Geometry: see drawing. Coordinates: mm, zero at the bounding-box minimum. A direction names the side the tool comes from. Coordinates: 2 decimals unless noted, no trailing zeros. Loops run counter-clockwise (first coordinate to the right, second up) from the corner with the lowest first, then second, coordinate; pieces in that order, holes last. Notation, with made-up numbers: (21.25, 64.5) -> (43.25, 64.5) arc R33 cw to (43.25, 103.5) -> close; hole circle Ø8 at (-26, 14). An arc over 180 degrees is marked (long way). Put each result on its own line as item: value. Start each with the question number.
1) Cut plane C-C (y = 0.75). Return the cut outline in (x, z), plus the area to 3 significant figures.
2) Material intervals for L1, parallel to X at y = 3.75, z = 15.75 (1 decimal); L2, parallel to X at y = 6, z = 16.25 (1 decimal); L3, parallel to X at y = 3, z = 18.75 (1 decimal), sorted ascending.
3) Pull-direction query (X, two-part tool) for the marked faces 1, 2 and 3; classes: pulls with the +X half, pulls with the -X half, needs draft (parallel to the pull), parting line crosses it, or undercut.
4) Set-up query: the marked faces 4, 5 and 6. Return all of +Z, -Z, +X, -X, +Y, -Y with unobstructed straight access to the full face (end or side cutting, diameter ignored); none if empty.
5) Cut plane A-A (x = 29). Return the cut outline in (y, z).
6) Cut plane D-D (x = 23). Return the cut outline in (y, z), plus the area to 3 significant figures.
7) Cut plane B-B (z = 7.75). Return the cut outline in (x, y).
8) Contact query for flat-ended pins moving along their axis: P1, Ø3, axis at x = 28.36, z = 15.13, coming from the +Y side; P2, Ø3.5, axis at x = 25, y = 4, coming from the -Z side; P3, Ø1, axis at y = 2.5, z = 4, coming from the -X side (1 decimal); P4, Ø1, axis at y = 1.5, z = 8, coming from the -X side (1 decimal). Output: stop coordinate, or through.
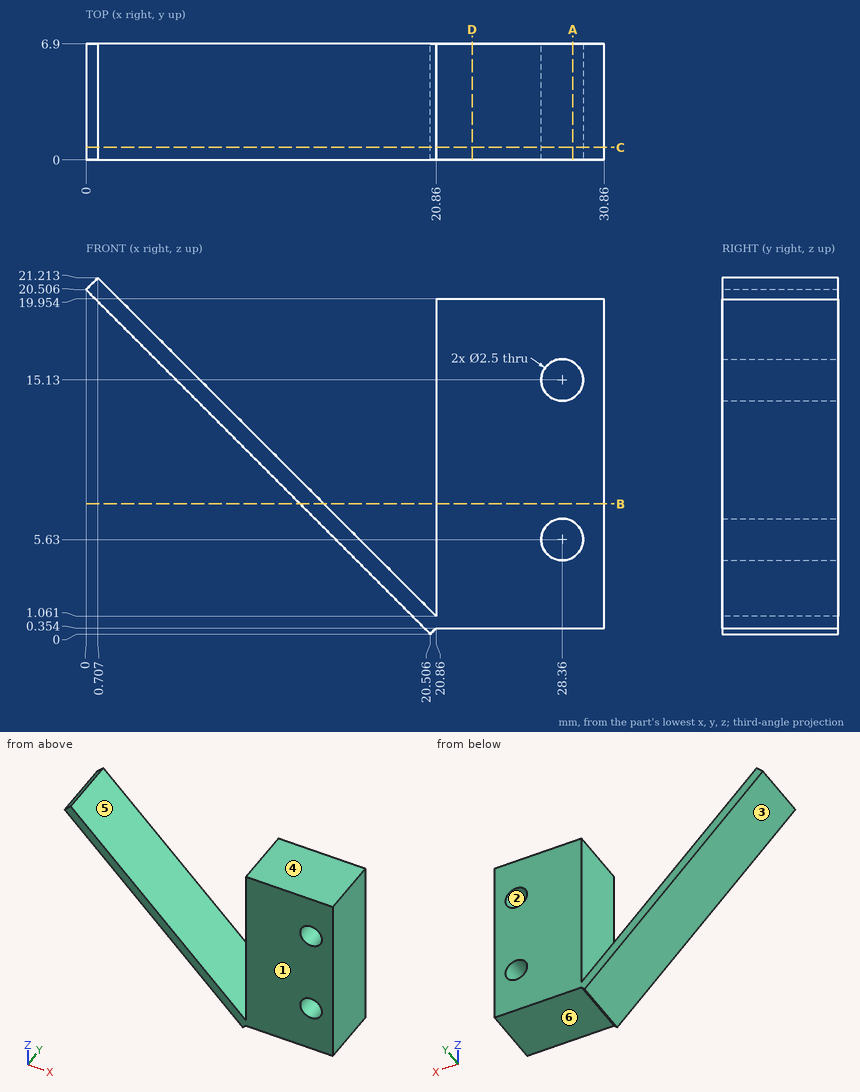
Results found:
1. outline: (0, 20.51) -> (20.51, 0) -> (20.86, 0.35) -> (30.86, 0.35) -> (30.86, 19.95) -> (20.86, 19.95) -> (20.86, 1.06) -> (0.71, 21.21) -> close; hole circle Ø2.5 at (28.36, 5.63); hole circle Ø2.5 at (28.36, 15.13)
1. area: 215 mm2
2. L1: x = 4.8 to 6.2, 20.9 to 27.3, 29.4 to 30.9
2. L2: x = 4.3 to 5.7, 20.9 to 27.8, 28.9 to 30.9
2. L3: x = 1.8 to 3.2, 20.9 to 30.9
3. face 1: needs draft
3. face 2: undercut
3. face 3: pulls with the -X half
4. face 4: +Z, +X, +Y, -Y
4. face 5: +Z, +Y, -Y
4. face 6: -Z, +X, +Y, -Y
5. outline: (0, 0.35) -> (6.9, 0.35) -> (6.9, 4.56) -> (0, 4.56) -> close; (0, 6.7) -> (6.9, 6.7) -> (6.9, 14.06) -> (0, 14.06) -> close; (0, 16.2) -> (6.9, 16.2) -> (6.9, 19.95) -> (0, 19.95) -> close
6. outline: (0, 0.35) -> (6.9, 0.35) -> (6.9, 19.95) -> (0, 19.95) -> close
6. area: 135 mm2
7. outline: (12.76, 0) -> (14.17, 0) -> (14.17, 6.9) -> (12.76, 6.9) -> close; (20.86, 0) -> (30.86, 0) -> (30.86, 6.9) -> (20.86, 6.9) -> close
8. P1: stops at y = 6.9
8. P2: stops at z = 0.35
8. P3: stops at x = 16
8. P4: stops at x = 12
